from build123d import *

# Parameters (mm, degrees)
F0_W     = 990.6
F0_H     = 152.4
F1_DEPTH = 2336.8
F3_DEPTH = 25.4
F5_DEPTH = 25.4
F7_DEPTH = 2387.6


with BuildPart() as f1:
    # F0 (on Top) → F1 (new body)
    with BuildSketch(Plane.XY):
        with Locations((0, 104.140009)):
            Rectangle(F0_W, F0_H)
    extrude(amount=F1_DEPTH)

    # F2 (on face) → F3 (join)
    with BuildSketch(Plane.XY.offset(2336.8)):
        with BuildLine():
            Line((-419.1, 104.140009), (-419.1, 129.540009))
            ThreePointArc((-419.1, 129.540009), (-437.060512, 122.100521), (-444.5, 104.140009))
            Line((-444.5, 104.140009), (-419.1, 104.140009))
        make_face()
        with BuildLine():
            ThreePointArc((-393.7, 104.140009), (-401.139488, 122.100521), (-419.1, 129.540009))
            Line((-419.1, 129.540009), (-419.1, 104.140009))
            Line((-419.1, 104.140009), (-444.5, 104.140009))
            ThreePointArc((-444.5, 104.140009), (-419.1, 78.740009), (-393.7, 104.140009))
        make_face()
    extrude(amount=F3_DEPTH)

    # F4 (on face) → F5 (join)
    with BuildSketch(Plane(origin=(0, 0, 0), x_dir=(1, 0, 0), z_dir=(0, 0, -1))):
        with BuildLine():
            Line((-419.1, -104.140009), (-419.1, -78.740009))
            ThreePointArc((-419.1, -78.740009), (-437.060512, -86.179497), (-444.5, -104.140009))
            Line((-444.5, -104.140009), (-419.1, -104.140009))
        make_face()
        with BuildLine():
            ThreePointArc((-393.7, -104.140009), (-401.139488, -86.179497), (-419.1, -78.740009))
            Line((-419.1, -78.740009), (-419.1, -104.140009))
            Line((-419.1, -104.140009), (-444.5, -104.140009))
            ThreePointArc((-444.5, -104.140009), (-419.1, -129.540009), (-393.7, -104.140009))
        make_face()
    extrude(amount=F5_DEPTH)

    # F6 (on face) → F7 (cut)
    with BuildSketch(Plane.XY.offset(2336.8)):
        with BuildLine():
            Line((-495.3, 27.940009), (-419.1, 27.940009))
            ThreePointArc((-419.1, 27.940009), (-472.981537, 50.258472), (-495.3, 104.140009))
            Line((-495.3, 104.140009), (-495.3, 27.940009))
        make_face()
        with BuildLine():
            ThreePointArc((-495.3, 104.140009), (-472.981537, 158.021546), (-419.1, 180.340009))
            Line((-419.1, 180.340009), (-495.3, 180.340009))
            Line((-495.3, 180.340009), (-495.3, 104.140009))
        make_face()
    extrude(amount=-F7_DEPTH, mode=Mode.SUBTRACT)


solid = f1.part
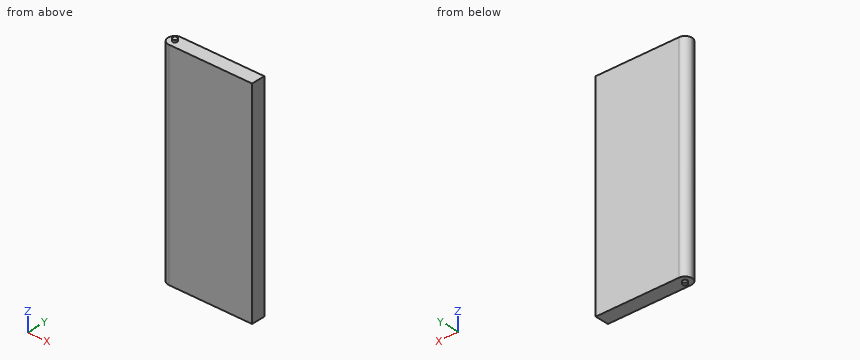
Verification items for the finished model (mm, model axes). Give positions to 0.01 mm unless a question says otherwise; leave off trailing zeros. Write each loop counter-clockwise with the first axis right and the second up, starting at its lowest first coordinate (ties: lowest second). Pieces come first, ordered by that corner, then holes.
(1) Material ranges on line 1 (Z direction, x = -216, y = 119.5); line 2 (X direction, y = 106.5, z = 518.5); line 3 (X direction, y = 99.5, z = 568), recorded low to high.
(2) Gauge pin test, flat ends, axial feed: pin 1 (4 mm diameter, centred on x = -365, y = 47.5, fed in from +Z); pin 2 (4 mm diameter, centred on x = -96, y = 58, fed in from -Z); pin 3 (2 mm diameter, centred on y = 135.5, z = 1408.5, fed in from -X). Record the tip position at first contact, or that the pin passes through.
(3) Cross-section at A-A (z = 947). Enter the section's corners in (x, y).
(4) Cross-section at B-B (x = -131.5). Enter the section's corners in (y, z).
Worked out:
1. line 1: z = 0 to 2336.8
1. line 2: x = -495.26 to 495.3
1. line 3: x = -495.16 to 495.3
2. pin 1: stops at z = 2336.8
2. pin 2: stops at z = 0
2. pin 3: stops at x = -488.99
3. outline: (-495.3, 104.14) arc R76.2 ccw to (-419.1, 27.94) - (495.3, 27.94) - (495.3, 180.34) - (-419.1, 180.34) arc R76.2 ccw to start
4. outline: (27.94, 0) - (180.34, 0) - (180.34, 2336.8) - (27.94, 2336.8) - close
